```python
from build123d import *

# Parameters (mm, degrees)
SKETCH1_W           = 165.1
SKETCH1_H           = 292.1
BOSS_EXTRUDE1_DEPTH = 3.175
FILLET1_R           = 50.8
SKETCH2_R           = 14.2875
CUT_EXTRUDE1_DEPTH  = 7.35
SKETCH4_R           = 3.175
CUT_EXTRUDE3_DEPTH  = 7.35
SKETCH5_R           = 9.525
SKETCH5_R_2         = 2.5527
CUT_EXTRUDE4_DEPTH  = 7.35


with BuildPart() as part:
    # Sketch1 → Boss-Extrude1 (new body, symmetric)
    with BuildSketch(Plane(origin=(0, 0, 0), x_dir=(0, 0, -1), z_dir=(1, 0, 0))):
        Rectangle(SKETCH1_W, SKETCH1_H)
    extrude(amount=BOSS_EXTRUDE1_DEPTH, both=True)

    # Fillet1
    fillet1_edges = [part.edges().sort_by_distance(p)[0] for p in [
        (0, -146.05, -82.55),
        (0, -146.05, 82.55),
        (0, 146.05, 82.55),
        (0, 146.05, -82.55),
    ]]
    fillet(fillet1_edges, radius=FILLET1_R)

    # Sketch2 → Cut-Extrude1 (cut, through all)
    with BuildSketch(Plane.ZY.offset(3.175)):
        with Locations((31.75, -95.25)):
            Circle(SKETCH2_R)
        with Locations((-31.75, 95.25)):
            Circle(SKETCH2_R)
    extrude(amount=-CUT_EXTRUDE1_DEPTH, mode=Mode.SUBTRACT)

    # Sketch4 → Cut-Extrude3 (cut, through all)
    with BuildSketch(Plane(origin=(3.175, 0, 0), x_dir=(0, 0, -1), z_dir=(1, 0, 0))):
        with Locations((62.241799111, 9.91138566)):
            Circle(SKETCH4_R)
        with Locations((-13.750490704, 4.288940581)):
            Circle(SKETCH4_R)
    extrude(amount=-CUT_EXTRUDE3_DEPTH, mode=Mode.SUBTRACT)

    # Sketch5 → Cut-Extrude4 (cut, through all)
    with BuildSketch(Plane.ZY.offset(3.175)):
        with Locations((46.230164374, 61.162830951)):
            Circle(SKETCH5_R)
        with Locations((63.959364374, 78.892030951)):
            Circle(SKETCH5_R_2)
        with Locations((28.500964374, 43.433630951)):
            Circle(SKETCH5_R_2)
    extrude(amount=-CUT_EXTRUDE4_DEPTH, mode=Mode.SUBTRACT)


solid = part.part
```
Here's how the part is built. I have some questions about the finished solid (model axes, mm). Coordinates: 2 decimals unless noted, no trailing zeros. Write each loop counter-clockwise with the first axis right and the second up, starting at its lowest first coordinate (ties: lowest second). Pieces come first, ordered by that corner, then holes. Notation, with made-up numbers: (6, 6.5) -> (33, 6.5) arc R30 cw to (33, 44.5) -> close; hole circle Ø10 at (35, -7). An arc over 180 degrees is marked (long way). Use a Markdown table: item, result. Add a question column.
(1) We'd pull the mould along Z, two halves only. Please class faces 1 (the flat face through (0, -1, -82.55)), 2 (the cylindrical face through (-0.044, 130.774, 68.064)), 3 (the cylindrical face through (-0.04, 41.17, 29.68)): +Z half, -Z half, draft (parallel to the pull), parting line (faces both ways), or undercut.
(2) I'm going to push a flat-ended pin straight in: P1, Ø1.5, axis at x = 0.5, z = 60.5, coming from the +Y side. Where does the tip first touch, or does it pass through?
(3) Please list where these lines run through material, in increasing order: line 1 (Y direction, x = 2, z = 30.5); line 2 (Y direction, x = 2, z = 27.5); line 3 (Y direction, x = 0, z = -39).
(4) If we section it at B-B, the plane y = 121: Write out the boundary of the cut face in (x, z) (3 decimals), and give its area (3 significant figures).
(5) If we section it at A-A, the plane x = 1.25: State how many separate pieces and enclosed holes the cut face has, and give its area (3 significant figures).
Outcome:
| question | item | result |
|---|---|---|
| 1 | face 1 | -Z half |
| 1 | face 2 | +Z half |
| 1 | face 3 | undercut |
| 2 | P1 | stops at y = 137.64 |
| 3 | line 1 | y = -146.05 to -109.48, -81.02 to 41.85, 45.02 to 146.05 |
| 3 | line 2 | y = -146.05 to -108.89, -81.61 to 41.09, 45.78 to 146.05 |
| 3 | line 3 | y = -145.53 to 82.94, 107.56 to 145.53 |
| 4 | outline | (-3.175, -75.54) -> (3.175, -75.54) -> (3.175, 75.54) -> (-3.175, 75.54) -> close |
| 4 | area | 959 mm^2 |
| 5 | separate pieces | 1 |
| 5 | enclosed holes | 7 |
| 5 | area | 44,300 mm^2 |
